Autodesk Fusion 360 part; units mm, degrees
sketch "Sketch1" plane through (0, 0, 0) normal (0, 0, 1) x (1, 0, 0)
  line L0 (1.7321, 2.75) -> (26.3431, 2.75)
  line L1 (26.3431, 2.75) -> (26.3431, -2.75)
  line L2 (26.3431, -2.75) -> (1.7321, -2.75)
  arc A0 (1.7321, 2.75) -> (1.7321, -2.75) centre (0, 0) ccw
  dimension "d1" = 6.5
  dimension "d2" = 5.5
  dimension "d3" = 24.611
  dimension "d4" = 5.5
sketch "Sketch2" plane through (0, 0, 0) normal (0, 0, 1) x (1, 0, 0)
sketch "Sketch3" plane through (0, 0, 0) normal (0, 0, 1) x (1, 0, 0)
extrude "Extrude1" add sketch "Sketch1" along normal blind 2.8
sketch "Sketch4" plane through (0, 0, 2.8) normal (0, 0, 1) x (-1, 0, 0)
  line L0 (-26.3431, -2.75) -> (-1.7321, -2.75)
  arc A0 (-1.7321, -2.75) -> (-1.7321, 2.75) centre (0, 0) ccw
  line L1 (-1.7321, 2.75) -> (-26.3431, 2.75)
  line L2 (-26.3431, 2.75) -> (-26.3431, -2.75)
  circle A1 centre (0, 0) radius 1.5
  dimension "d7" = 3
extrude "Extrude2" add sketch "Sketch4" along normal blind 10 contours A1
fillet "Fillet1" radius 1 4 edges at (14.0376, -2.75, 2.8) (14.0376, 2.75, 2.8) (14.0376, 2.75, 0) (14.0376, -2.75, 0)
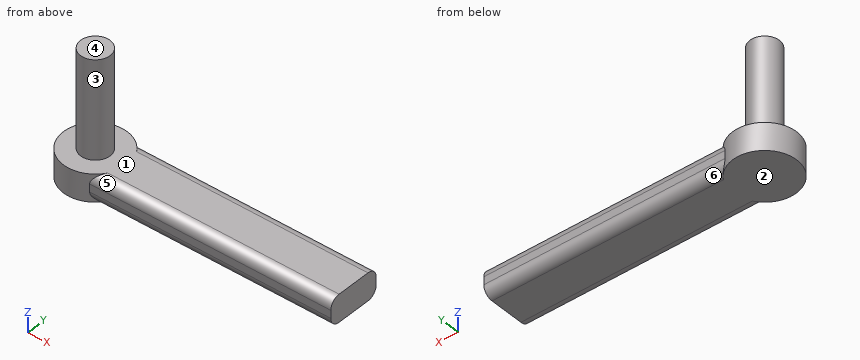
Could you check a few things on this model? Use its own coordinates, in mm. Face numbers are marked on the shaded views. A direction names the side the tool comes from. Round coordinates to 2 decimals unless told otherwise and drop trailing zeros. Write each loop counter-clockwise with the first axis right and the second up, starting at its lowest first coordinate (ties: lowest second). Pieces come first, ordered by that corner, then holes. Notation, with made-up numbers: (-33, 76) - (-9, 76) arc R12 ccw to (-9, 90) - close; hole circle Ø10 at (17.5, 22.25). An arc over 180 degrees is marked (long way). Use a Markdown table: item, result.
Q1. For pin 1 (2 mm diameter, centred on y = 0.5, z = 9, fed in from +X); pin 2 (3.5 mm diameter, centred on x = 9.5, y = 0.5, fed in from +Z); pin 3 (1 mm diameter, centred on x = 7.5, z = 2, fed in from -Y), each with a flat end and sliding along its axis, tell me the tip position at first contact or that it passes through.
Output values:
| item | result |
|---|---|
| pin 1 | x = 1.5 |
| pin 2 | z = 2.8 |
| pin 3 | y = -2.75 |
Q2. I want a section at B-B (y = 2.25). List the corners of the cut face in (x, z) for me, plus the area to 3 significant figures.
Output values:
| item | result |
|---|---|
| outline | (-2.35, 0) - (2.35, 0) - (2.35, 0.13) - (26.34, 0.13) - (26.34, 2.67) - (2.35, 2.67) - (2.35, 2.8) - (-2.35, 2.8) - close |
| area | 73.9 mm2 |
Q3. Please list where these lines run through material, in increasing order: L1, parallel to Z at x = 5.5, y = -1.75; L2, parallel to Y at x = 6.5, z = 1.5; L3, parallel to X at y = 0, z = 3.
Output values:
| item | result |
|---|---|
| L1 | 0 to 2.8 |
| L2 | -2.75 to 2.75 |
| L3 | -1.5 to 1.5 |
Q4. Thinking about a two-plate mould opening in Z: for the marked faces 1, 2 and 3, which applies, released by +Z, released by -Z, zero draft, split by the parting line, or undercut?
Output values:
| item | result |
|---|---|
| face 1 | released by +Z |
| face 2 | released by -Z |
| face 3 | zero draft |
Q5. I want a section at C-C (z = 6.25). List the corners of the cut face in (x, y) for me.
Output values:
| item | result |
|---|---|
| outline | circle Ø3 at (0, 0) |
Q6. I want a section at D-D (x = 2.25). List the corners of the cut face in (y, z) for me, plus the area to 3 significant figures.
Output values:
| item | result |
|---|---|
| outline | (-2.75, 1) arc R1 ccw to (-2.35, 0.2) - (-2.35, 0) - (2.35, 0) - (2.35, 0.2) arc R1 ccw to (2.75, 1) - (2.75, 1.8) arc R1 ccw to (2.35, 2.6) - (2.35, 2.8) - (-2.35, 2.8) - (-2.35, 2.6) arc R1 ccw to (-2.75, 1.8) - close |
| area | 14.7 mm2 |
Q7. I want a section at A-A (x = 5.5). List the corners of the cut face in (y, z) for me.
Output values:
| item | result |
|---|---|
| outline | (-2.75, 1) arc R1 ccw to (-1.75, 0) - (1.75, 0) arc R1 ccw to (2.75, 1) - (2.75, 1.8) arc R1 ccw to (1.75, 2.8) - (-1.75, 2.8) arc R1 ccw to (-2.75, 1.8) - close |
Q8. For the marked faces 4, 5 and 6, which set-ups out of +Z, -Z, +X, -X, +Y, -Y let a thin tool reach every point of the face, with its end or its side?
Output values:
| item | result |
|---|---|
| face 4 | +Z, +X, -X, +Y, -Y |
| face 5 | +Z, +X, -Y |
| face 6 | -Z, +X, +Y |
